from build123d import *

# Parameters (mm, degrees)
F1_DEPTH = 1.2
F2_W     = 4.9
F2_H     = 6.2
F2_W_2   = 4.6
F2_H_2   = 16.2
F2_W_3   = 0.3
F2_H_3   = 24.4
F4_DEPTH = 2.2
F2_W_4   = 12
F2_H_4   = 16
F5_DEPTH = 2.4
F2_W_5   = 5.2
F2_H_5   = 7.8
F6_DEPTH = 1


with BuildPart() as f1:
    # F0 (on Right) → F1 (new body)
    with BuildSketch(Plane.YZ):
        Polygon((74.45, 0), (74.45, 46), (68.05, 46), (68.05, 49), (53.05, 49.527473), (53.05, 46), (50.85, 46), (50.85, 49.604835), (39.35, 50.009231), (39.35, 47.8), (37.15, 47.8), (37.15, 50.086593), (22.55, 50.6), (22.55, 47.8), (20.35, 47.8), (20.35, 48.9), (-24.45, 48.9), (-24.45, 47.8), (-26.65, 47.8), (-26.65, 50.5), (-38.95, 50.054348), (-38.95, 47.8), (-41.15, 47.8), (-41.15, 49.974638), (-68.05, 49), (-68.05, 46), (-74.45, 46), (-74.45, 0), align=None)
    extrude(amount=F1_DEPTH)

    # F2 (on face) → F4 (join)
    with BuildSketch(Plane(origin=(0, 0, 0), x_dir=(0, -1, 0), z_dir=(-1, 0, 0))):
        with Locations((71, 34.9)):
            Rectangle(F2_W, F2_H)
        with Locations((72.15, 18)):
            Rectangle(F2_W_2, F2_H_2)
        with Locations((74.6, 18)):
            Rectangle(F2_W_3, F2_H_2)
        with Locations((-8.7, 13.2)):
            Rectangle(F2_W, F2_H_3)
    extrude(amount=F4_DEPTH)

    # F2 (on face) → F5 (join)
    with BuildSketch(Plane(origin=(0, 0, 0), x_dir=(0, -1, 0), z_dir=(-1, 0, 0))):
        with Locations((55.55, 39.8)):
            Rectangle(F2_W_4, F2_H_4)
    extrude(amount=F5_DEPTH)

    # F2 (on face) → F6 (join)
    with BuildSketch(Plane(origin=(0, 0, 0), x_dir=(0, -1, 0), z_dir=(-1, 0, 0))):
        with Locations((50.35, 21.4)):
            Rectangle(F2_W_5, F2_H_5)
        with Locations((59.55, 21.4)):
            Rectangle(F2_W_5, F2_H_5)
    extrude(amount=F6_DEPTH)


solid = f1.part
The model under review builds one solid part; all positions refer to its coordinate system, in mm. A direction names the side the tool comes from. Coordinates: 2 decimals unless noted, no trailing zeros. Order: outer loops, then holes, each group sorted by start corner. A loop starts at its lowest first (then second) coordinate and runs counter-clockwise, first axis right, second up. Notation, with made-up numbers: (-24.75, 17.25) -> (-6.75, 17.25) arc R19 ccw to (-6.75, 44.25) -> close; hole circle Ø3 at (37, -37.75). An arc over 180 degrees is marked (long way). Answer in a Markdown table with one row per item.
(1) Consider section B-B (z = 36). Write out the cut boundary in (x, y), plus the area to 3 significant figures.
Answers:
| item | result |
|---|---|
| outline | (-2.4, -61.55) -> (0, -61.55) -> (0, -68.55) -> (-2.2, -68.55) -> (-2.2, -73.45) -> (0, -73.45) -> (0, -74.45) -> (1.2, -74.45) -> (1.2, 74.45) -> (0, 74.45) -> (0, -49.55) -> (-2.4, -49.55) -> close |
| area | 218 mm² |
(2) Consider section A-A (z = 14). Write out the cut boundary in (x, y).
Answers:
| item | result |
|---|---|
| outline | (-2.2, -74.75) -> (0, -74.75) -> (0, -74.45) -> (1.2, -74.45) -> (1.2, 74.45) -> (0, 74.45) -> (0, 11.15) -> (-2.2, 11.15) -> (-2.2, 6.25) -> (0, 6.25) -> (0, -69.85) -> (-2.2, -69.85) -> close |
(3) Wall thickness on line 1 along Y through (x, z) = (-1.7, 20); line 2 along Y through (x, z) = (-0.95, 34); line 3 along X through (y, z) = (61.5, 25.5): over which ranges is each line inside the solid? List them lowest first.
Answers:
| item | result |
|---|---|
| line 1 | -74.75 to -69.85, 6.25 to 11.15 |
| line 2 | -73.45 to -68.55, -61.55 to -49.55 |
| line 3 | 0 to 1.2 |
(4) Consider section C-C (y = -28.5). Write out the cut boundary in (x, z), plus the area to 3 significant figures.
Answers:
| item | result |
|---|---|
| outline | (0, 0) -> (1.2, 0) -> (1.2, 50.43) -> (0, 50.43) -> close |
| area | 60.5 mm² |
(5) Machinability: for faces 4 (the flat face through (-1, -55, 47.8)), 5 (the flat face through (-1, -61.55, 40)), 6 (the flat face through (-1, -55, 31.8)), 7 (the flat face through (-1, -60, 21)), which of the approach directions +Z, -Z, +X, -X, +Y, -Y give a long, thin tool a straight path to every point of the face, cutting with its end or side? Answer none if there is none.
Answers:
| item | result |
|---|---|
| face 4 | +Z, -X, +Y, -Y |
| face 5 | +Z, -X |
| face 6 | -X, +Y, -Y |
| face 7 | -Z, -X |
(6) The part is to be moulded in two halves that separate along Y. For faces 1 (the flat face through (-2.2, 9, 13)), 2 (the flat face through (-1, -50, 21)), 3 (the flat face through (-1, -49.55, 40)), say which applies: +Y half, -Y half, draft (parallel to the pull), parting line (faces both ways), or undercut.
Answers:
| item | result |
|---|---|
| face 1 | draft |
| face 2 | undercut |
| face 3 | +Y half |
(7) Insertion check: pin 1 (8 mm diameter, centred on y = 17, z = 38.5, fed in from -X); pin 2 (1.1 mm diameter, centred on x = -1, y = -73.5, fed in from -Z); pin 3 (1.1 mm diameter, centred on x = -0.5, z = 17.5, fed in from +Y); pin 4 (1 mm diameter, centred on x = 0.5, y = -70, fed in from +Z). Each pin has a flat end and moves straight along its axis. Give the tip position at first contact, or say it passes through.
Answers:
| item | result |
|---|---|
| pin 1 | x = 0 |
| pin 2 | z = 9.9 |
| pin 3 | y = 74.45 |
| pin 4 | z = 46 |
(8) Consider section D-D (y = -6.5). Write out the cut boundary in (x, z).
Answers:
| item | result |
|---|---|
| outline | (0, 0) -> (1.2, 0) -> (1.2, 48.9) -> (0, 48.9) -> close |
